from build123d import *

# Parameters (mm, degrees)
F1_DEPTH = 12
F2_DEPTH = 43
F4_DEPTH = 22
F5_R     = 2
F6_DEPTH = 15
F7_DEPTH = 15


with BuildPart() as f1:
    # F0 (on Top) → F1 (new body)
    with BuildSketch(Plane.XY):
        with BuildLine():
            ThreePointArc((2.394141, -6.577848), (5.734064, -4.015035), (7, 0))
            ThreePointArc((7, 0), (4.949747, 4.949747), (0, 7))
            Line((0, 7), (0, 5.6))
            ThreePointArc((0, 5.6), (3.959798, 3.959798), (5.6, 0))
            ThreePointArc((5.6, 0), (4.587251, -3.212028), (1.915313, -5.262279))
            Line((1.915313, -5.262279), (2.394141, -6.577848))
        make_face()
        with BuildLine():
            ThreePointArc((2.394141, -6.577848), (-6.893654, -1.215537), (0, 7))
            Line((0, 7), (0, 14))
            ThreePointArc((0, 14), (-13.787309, -2.431074), (4.788282, -13.155697))
            Line((4.788282, -13.155697), (2.394141, -6.577848))
        make_face()
    extrude(amount=F1_DEPTH)

    # F0 (on Top) → F2 (join)
    with BuildSketch(Plane.XY):
        with BuildLine():
            Line((0, 0), (0, 5.6))
            ThreePointArc((0, 5.6), (-5.514923, -0.97243), (1.915313, -5.262279))
            Line((1.915313, -5.262279), (0, 0))
        make_face()
        with BuildLine():
            ThreePointArc((5.6, 0), (3.959798, 3.959798), (0, 5.6))
            Line((0, 5.6), (0, 0))
            Line((0, 0), (1.915313, -5.262279))
            ThreePointArc((1.915313, -5.262279), (4.587251, -3.212028), (5.6, 0))
        make_face()
        with BuildLine():
            Line((0, 5.6), (0, 7))
            ThreePointArc((0, 7), (-6.893654, -1.215537), (2.394141, -6.577848))
            Line((2.394141, -6.577848), (1.915313, -5.262279))
            ThreePointArc((1.915313, -5.262279), (-5.514923, -0.97243), (0, 5.6))
        make_face()
        with BuildLine():
            ThreePointArc((2.394141, -6.577848), (5.734064, -4.015035), (7, 0))
            ThreePointArc((7, 0), (4.949747, 4.949747), (0, 7))
            Line((0, 7), (0, 5.6))
            ThreePointArc((0, 5.6), (3.959798, 3.959798), (5.6, 0))
            ThreePointArc((5.6, 0), (4.587251, -3.212028), (1.915313, -5.262279))
            Line((1.915313, -5.262279), (2.394141, -6.577848))
        make_face()
    extrude(amount=F2_DEPTH)

    # F3 (on face) → F4 (join)
    with BuildSketch(Plane.XY.offset(43)):
        Polygon((7, 0), (3.5, 6.062178), (-3.5, 6.062178), (-7, 0), (-3.5, -6.062178), (3.5, -6.062178), align=None)
    extrude(amount=F4_DEPTH)

    # F5 (on face) → F6 (cut)
    with BuildSketch(Plane.XY.offset(65)):
        Circle(F5_R)
    extrude(amount=-F6_DEPTH, mode=Mode.SUBTRACT)

    # F0 (on Top) → F7 (cut)
    with BuildSketch(Plane.XY):
        with BuildLine():
            Line((0, 0), (0, 5.6))
            ThreePointArc((0, 5.6), (-5.514923, -0.97243), (1.915313, -5.262279))
            Line((1.915313, -5.262279), (0, 0))
        make_face()
        with BuildLine():
            ThreePointArc((5.6, 0), (3.959798, 3.959798), (0, 5.6))
            Line((0, 5.6), (0, 0))
            Line((0, 0), (1.915313, -5.262279))
            ThreePointArc((1.915313, -5.262279), (4.587251, -3.212028), (5.6, 0))
        make_face()
    extrude(amount=F7_DEPTH, mode=Mode.SUBTRACT)


solid = f1.part
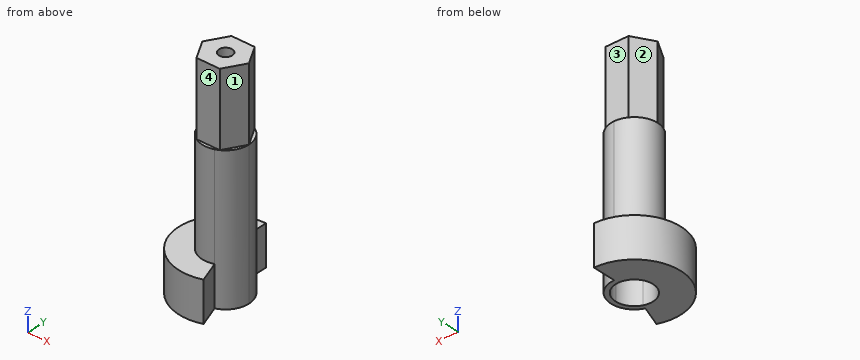
CAD build for the part. Positions are in the model's coordinates, mm. Face numbers are marked on the shaded views. A direction names the side the tool comes from. Coordinates: 2 decimals unless noted, no trailing zeros. Write each loop counter-clockwise with the first axis right and the second up, starting at its lowest first coordinate (ties: lowest second). Pieces come first, ordered by that corner, then holes. Notation, with made-up numbers: M -9.75,-19 L 26.25,-19 A21 ccw 26.25,2 Z; hole C 39,81.25 d5. An arc over 180 degrees is marked long. Answer as a JSON object with one key per item and string values. Group by question number.
1) Wall check: line 1 (Y direction, x = 0, z = 59.25); line 2 (Z direction, x = -11.5, y = -2.5); line 3 (Z direction, x = 2.75, y = -6.25). Give the ranges that are in metal, low to high. Write a range as from..to.
2) Saw through at A-A (z = 10.5). Write the cut outline in (x, y).
3) Saw through at D-D (y = 8). Write the cut outline in (x, z), plus the area to 3 significant figures.
4) Saw through at B-B (x = 1). Write the cut outline in (y, z).
5) Tool access for the marked faces 1, 2, 3 and 4: list every direction of +Z, -Z, +X, -X, +Y, -Y with a clear straight run to the whole face (end or side of a thin tool).
6) Pin check, flat tips, straight feed: pin 1 Ø3.5 at (x, z) = (0.5, 58) entering from +Y; pin 2 Ø1.7 at (x, y) = (5.5, -4.5) entering from +Z; pin 3 Ø2 at (x, z) = (3, 7.5) entering from +Y. Stop position of each tip, or through.
7) Saw through at C-C (z = 18). Write the cut outline in (x, y).
Values follow:
{
 "1": {"line 1": "y = -6.06..-2, 2..6.06", "line 2": "z = 0..12", "line 3": "z = 0..43"},
 "2": {"outline": "M 0,7 L 0,14 A14 ccw long 4.79,-13.16 L 2.39,-6.58 A7 ccw 7,0 A7 ccw Z; hole M 1.92,-5.26 A5.6 ccw 5.6,0 A5.6 ccw long Z"},
 "3": {"outline": "M -11.49,0 L 0,0 L 0,12 L -11.49,12 Z", "area": "138 mm2"},
 "4": {"outline": "M -13.96,0 L -5.51,0 L -5.51,15 L 5.51,15 L 5.51,0 L 6.93,0 L 6.93,43 L 6.06,43 L 6.06,65 L 1.73,65 L 1.73,50 L -1.73,50 L -1.73,65 L -6.06,65 L -6.06,43 L -6.93,43 L -6.93,12 L -13.96,12 Z"},
 "5": {"face 1": "+Z, +X, -Y", "face 2": "+Z, -X, +Y", "face 3": "+Z, +X, -X, +Y", "face 4": "+Z, +X, -X, -Y"},
 "6": {"pin 1": "stops at y = 6.06", "pin 2": "stops at z = 43", "pin 3": "stops at y = 6.71"},
 "7": {"outline": "M 0,7 A7 ccw long 7,0 A7 ccw Z"}
}
